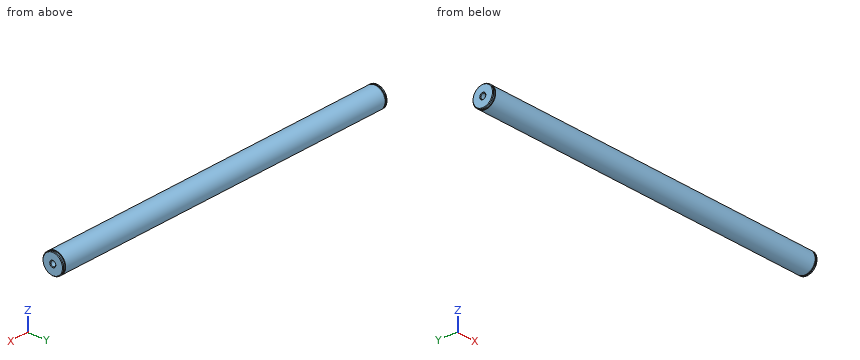
```python
from build123d import *

# Parameters (mm, degrees)
SKETCH1_R           = 11.176
BOSS_EXTRUDE1_DEPTH = 193.3575
CUT_EXTRUDE1_START  = -1.778
SKETCH2_OUTSIDE_W   = 101.952
SKETCH2_OUTSIDE_H   = 101.952
SKETCH2_OUTSIDE_R   = 10.541
CUT_EXTRUDE1_DEPTH  = 1.27
SKETCH3_R           = 2.667
CUT_EXTRUDE2_DEPTH  = 25.4
CHAMFER1_SIZE       = 0.635


with BuildPart() as part:
    # Sketch1 → Boss-Extrude1 (new, symmetric)
    with BuildSketch(Plane(origin=(0, 0, 0), x_dir=(0, 0, -1), z_dir=(1, 0, 0))):
        Circle(SKETCH1_R)
    extrude(amount=BOSS_EXTRUDE1_DEPTH, both=True)

    # Sketch2 outside → Cut-Extrude1 (cut)
    with BuildSketch(Plane.ZY.offset(193.3575).offset(CUT_EXTRUDE1_START)):
        Rectangle(SKETCH2_OUTSIDE_W, SKETCH2_OUTSIDE_H)
        Circle(SKETCH2_OUTSIDE_R, mode=Mode.SUBTRACT)
    cut_extrude1 = extrude(amount=-CUT_EXTRUDE1_DEPTH, mode=Mode.SUBTRACT)

    # Sketch3 → Cut-Extrude2 (cut)
    with BuildSketch(Plane.ZY.offset(193.3575)):
        Circle(SKETCH3_R)
    cut_extrude2 = extrude(amount=-CUT_EXTRUDE2_DEPTH, mode=Mode.SUBTRACT)

    # Mirror1: Cut-Extrude1, Cut-Extrude2 across plane
    add(cut_extrude1.mirror(Plane(origin=(0, 0, 0), x_dir=(0, 0, 1), z_dir=(1, 0, 0))), mode=Mode.SUBTRACT)
    add(cut_extrude2.mirror(Plane(origin=(0, 0, 0), x_dir=(0, 0, 1), z_dir=(1, 0, 0))), mode=Mode.SUBTRACT)

    # Chamfer1
    chamfer1_edges = [part.edges().sort_by_distance(p)[0] for p in [
        (-193.3575, 0, 11.176),
        (-193.3575, 0, -2.667),
        (193.3575, 0, 11.176),
        (193.3575, 0, -2.667),
    ]]
    chamfer(chamfer1_edges, length=CHAMFER1_SIZE)


solid = part.part
```
Input: part model. Units: mm. Frame: model coordinates. Give positions to 0.01 mm unless a question says otherwise; leave off trailing zeros. Order: outer loops, then holes, each group sorted by start corner. A loop starts at its lowest first (then second) coordinate and runs counter-clockwise, first axis right, second up.
1. Section A-A on x = -127. Return the cut outline in (y, z), and give its area (3 significant figures).
Derived:
outline: circle Ø22.35 at (0, 0)
area: 392 mm2
2. Pin query (flat end, axial travel): pin 1 (8 mm diameter, centred on x = -141.5, y = -5.5, fed in from +Z); pin 2 (4.5 mm diameter, centred on y = 0, z = -0.5, fed in from -X); pin 3 (4.5 mm diameter, centred on y = 0, z = 0, fed in from +X). Return the tip coordinate at first contact, or that it passes through.
Derived:
pin 1: stops at z = 11.07
pin 2: stops at x = -192.81
pin 3: stops at x = 167.96
3. Material intervals for L1, parallel to Y at x = 174, z = -0.25; L2, parallel to Z at x = 175, y = 2.25; L3, parallel to X at y = -6, z = -9, sorted ascending.
Derived:
L1: y = -11.17 to -2.66, 2.66 to 11.17
L2: z = -10.95 to -1.43, 1.43 to 10.95
L3: x = -193.08 to -191.58, -190.31 to 190.31, 191.58 to 193.08
